Check sheet for the modelled part. Datum: model origin and axes. Units: mm. Face numbers are marked on the shaded views. A direction names the side the tool comes from. Round coordinates to 2 decimals unless told otherwise and drop trailing zeros. Order: outer loops, then holes, each group sorted by start corner. A loop starts at its lowest first (then second) coordinate and runs counter-clockwise, first axis right, second up. Notation, with made-up numbers: (-14, -13) -> (17, -13) arc R15 ccw to (17, -2) -> close; hole circle Ø6 at (41, 12). An arc over 180 degrees is marked (long way). Answer in a Markdown table with one row per item. Add a question column.
1. Sectioned sample at A-A, the plane z = 1. Record the boundary of the cut face in (x, y), then the cut area to 3 significant figures.
2. Depth check by flat-ended pin: P1, Ø0.9, axis at x = 0, y = 0, coming from the +Z side; P2, Ø1.5, axis at y = 0, z = -4, coming from the -X side. Enter the tip coordinate at first touch or a pass-through.
3. Sectioned sample at B-B, the plane y = 0. Record the boundary of the cut face in (x, z).
4. Sectioned sample at C-C, the plane z = -2. Record the boundary of the cut face in (x, y), then the cut area to 3 significant figures.
5. Draft check along Y on the marked faces 1, 2, 3 and 4. Enter one of: +Y half, -Y half, draft (parallel to the pull), parting line (faces both ways), or undercut.
6. Access from +Z, -Z, +X, -X, +Y, -Y to the whole of each face (thin tool, end or side, straight path). Record for the marked faces 5 and 6.
7. Sectioned sample at D-D, the plane z = -7. Record the boundary of the cut face in (x, y).
8. Material ranges on L1, parallel to Z at x = 0.75, y = 1.75; L2, parallel to Z at x = 0, y = -0.5; L3, parallel to Y at x = 0, z = -4.5, recorded low to high. Write a range as from..to.
```python
from build123d import *

# Parameters (mm, degrees)
PAD_DEPTH    = 3
SKETCH001_R  = 1.5
POCKET_DEPTH = 4
SKETCH004_R  = 1.5
PAD001_DEPTH = 5


with BuildPart() as part:
    # Sketch → Pad (new body, symmetric)
    with BuildSketch(Plane.XY):
        Polygon((2.6, 1.501111), (0, 3.002221), (-2.6, 1.501111), (-2.6, -1.501111), (0, -3.002221), (2.6, -1.501111), align=None)
    extrude(amount=PAD_DEPTH, both=True)

    # Sketch001 (on Face8 of Pad) → Pocket (cut)
    with BuildSketch(Plane.XY.offset(3)):
        Circle(SKETCH001_R)
    extrude(amount=-POCKET_DEPTH, mode=Mode.SUBTRACT)

    # Sketch004 (on Face4 of Pocket) → Pad001 (join)
    with BuildSketch(Plane(origin=(0, 0, -3), x_dir=(1, 0, 0), z_dir=(0, 0, -1))):
        Circle(SKETCH004_R)
    extrude(amount=PAD001_DEPTH)

    # Sketch006 → Groove (revolve, cut)
    with BuildSketch(Plane.YZ):
        Polygon((1.8, 3.75), (4.8, 3.75), (4.8, -3.75), (1.8, -3.75), (3.55, -2), (3.55, 2), align=None)
    revolve(axis=Axis((0, 0, 0), (0, 0, 1)), mode=Mode.SUBTRACT)


solid = part.part
```
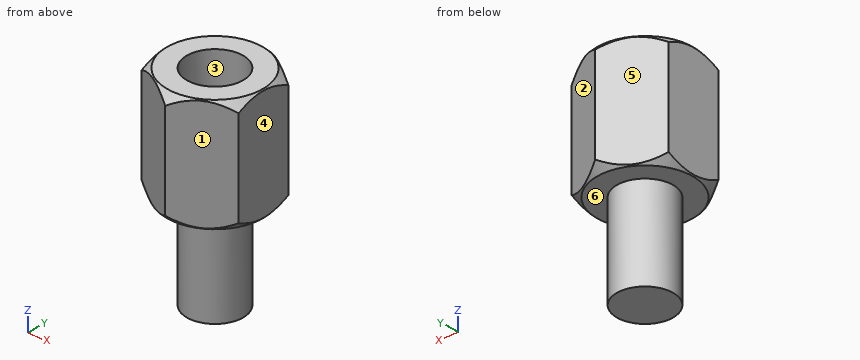
Answer key:
| question | item | result |
|---|---|---|
| 1 | outline | (-2.6, -1.5) -> (0, -3) -> (2.6, -1.5) -> (2.6, 1.5) -> (0, 3) -> (-2.6, 1.5) -> close; hole circle Ø3 at (0, 0) |
| 1 | area | 16.3 mm² |
| 2 | P1 | stops at z = -1 |
| 2 | P2 | stops at x = -1.5 |
| 3 | outline | (-2.6, -2.95) -> (-2.55, -3) -> (-1.5, -3) -> (-1.5, -8) -> (1.5, -8) -> (1.5, -3) -> (2.55, -3) -> (2.6, -2.95) -> (2.6, 2.95) -> (2.55, 3) -> (1.5, 3) -> (1.5, -1) -> (-1.5, -1) -> (-1.5, 3) -> (-2.55, 3) -> (-2.6, 2.95) -> close |
| 4 | outline | (-2.6, -1.5) -> (0, -3) -> (2.6, -1.5) -> (2.6, 1.5) -> (0, 3) -> (-2.6, 1.5) -> close |
| 4 | area | 23.4 mm² |
| 5 | face 1 | -Y half |
| 5 | face 2 | +Y half |
| 5 | face 3 | undercut |
| 5 | face 4 | draft |
| 6 | face 5 | +Z, -Z, -X, +Y |
| 6 | face 6 | -Z |
| 7 | outline | circle Ø3 at (0, 0) |
| 8 | L1 | z = -3..3 |
| 8 | L2 | z = -8..-1 |
| 8 | L3 | y = -1.5..1.5 |
